Read the model definition and answer for the solid it produces. Units are mm, in the model's axes. Face numbers are marked on the shaded views. A direction names the side the tool comes from. Coordinates: 2 decimals unless noted, no trailing zeros. Write each loop counter-clockwise with the first axis right and the second up, starting at its lowest first coordinate (ties: lowest second). Pieces come first, ordered by that corner, then holes.
(1) Which of the six approach directions +Z, -Z, +X, -X, +Y, -Y give full straight-line access (tool end or side, diameter ignored) to the marked faces 1 and 2?
(2) Given pin 1 (3 mm diameter, centred on x = -10.5, y = -4.5, fed in from +Z); pin 2 (15 mm diameter, centred on x = 10, z = 563, fed in from -Y); pin 3 (3 mm diameter, centred on x = -12, y = -3, fed in from -Z), each flat-ended and moving along its own axis, determine where each tip first touches the part or whether it passes through.
(3) Section B-B on x = 13 is taken. Write down the section's boundary in (y, z) (3 decimals), then the cut area to 3 significant figures.
(4) Find the intervals of material crossed by probe 1 along Z at (x, y) = (0, 5.5); probe 2 along Z at (x, y) = (23, -2); probe 3 along X at (y, z) = (6.25, 342.9), in increasing order.
(5) Section A-A on y = -3 is taken. Write down the section's boundary in (x, z).
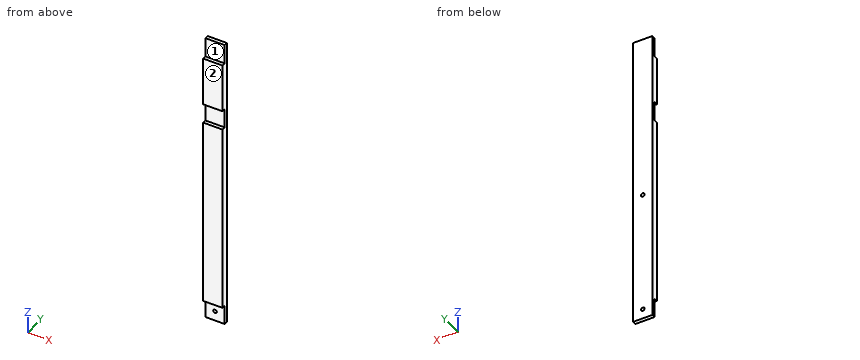
from build123d import *

# Parameters (mm, degrees)
F0_W     = 50.8
F0_H     = 19.05
F1_DEPTH = 774.7
F2_W     = 122.43557321
F2_H     = 50.8
F2_W_2   = 343.1604206562
F2_W_3   = 261.0546275973
F3_DEPTH = 25.4
F4_R     = 4.7625
F5_DEPTH = 25.4


# Not quite as in the source:
# - a feature names something its author has since deleted; it is built from what else it names


with BuildPart() as f1:
    # F0 (on Top) → F1 (new body)
    with BuildSketch(Plane.XY):
        Rectangle(F0_W, F0_H)
    extrude(amount=F1_DEPTH)

    # F2 (on Front) → F3 (cut)
    with BuildSketch(Plane.XZ):
        with Locations((22.4465244144, 25.4)):
            Rectangle(F2_W, F2_H)
        with Locations((-38.7818217278, 749.3)):
            Rectangle(F2_W_2, F2_H)
        with Locations((-37.622589618, 571.5)):
            Rectangle(F2_W_3, F2_H)
    extrude(amount=F3_DEPTH, mode=Mode.SUBTRACT)

    # F4 (on Front) → F5 (cut)
    with BuildSketch(Plane.XZ):
        with Locations((0, 25.4)):
            Circle(F4_R)
        with Locations((0, 342.9)):
            Circle(F4_R)
    extrude(amount=-F5_DEPTH, mode=Mode.SUBTRACT)


solid = f1.part
Response:
1. face 1: +Z, +X, -X, -Y
1. face 2: +Z, -Z, +X, -X, -Y
2. pin 1: stops at z = 723.9
2. pin 2: stops at y = 0
2. pin 3: stops at z = 50.8
3. outline: (-9.525, 50.8) - (0, 50.8) - (0, 0) - (9.525, 0) - (9.525, 774.7) - (0, 774.7) - (0, 723.9) - (-9.525, 723.9) - (-9.525, 596.9) - (0, 596.9) - (0, 546.1) - (-9.525, 546.1) - close
3. area: 13,300 mm2
4. probe 1: z = 0 to 20.64, 30.16 to 338.14, 347.66 to 774.7
4. probe 2: z = 50.8 to 546.1, 596.9 to 723.9
4. probe 3: x = -25.4 to -4.76, 4.76 to 25.4
5. outline: (-25.4, 50.8) - (25.4, 50.8) - (25.4, 546.1) - (-25.4, 546.1) - close; (-25.4, 596.9) - (25.4, 596.9) - (25.4, 723.9) - (-25.4, 723.9) - close
